For this review, take the finished solid that the model builds, in its own axes (mm). Give positions to 0.01 mm unless a question says otherwise; leave off trailing zeros. Loops run counter-clockwise (first coordinate to the right, second up) from the corner with the lowest first, then second, coordinate; pieces in that order, holes last. Notation, with made-up numbers: (57, 0.25) - (75, 0.25) arc R15 ccw to (75, 21.25) - close; hole circle Ø7 at (14.25, 68). An arc over 180 degrees is marked (long way). Answer as CSV lines item,"result".
from build123d import *

# Parameters (mm, degrees)
SKETCH1_R           = 2.6
BOSS_EXTRUDE1_DEPTH = 3.175


with BuildPart() as part:
    # Sketch1 → Boss-Extrude1 (new body)
    with BuildSketch(Plane(origin=(0, 0, 0), x_dir=(1, 0, 0), z_dir=(0, 1, 0))):
        Polygon((60, 0), (60, 20), (20, 60), (0, 60), (0, 0), align=None)
        with Locations((50, 10)):
            Circle(SKETCH1_R, mode=Mode.SUBTRACT)
        with Locations((10, 50)):
            Circle(SKETCH1_R, mode=Mode.SUBTRACT)
        with Locations((30, 10)):
            Circle(SKETCH1_R, mode=Mode.SUBTRACT)
        with Locations((10, 10)):
            Circle(SKETCH1_R, mode=Mode.SUBTRACT)
        with Locations((10, 30)):
            Circle(SKETCH1_R, mode=Mode.SUBTRACT)
    extrude(amount=BOSS_EXTRUDE1_DEPTH)


solid = part.part
1) Wall thickness on line 1 (X direction, y = 2, z = -10); line 2 (X direction, y = 2.45, z = -8.5); line 3 (Z direction, x = 50, y = 1.05): over which ranges is each line inside the solid? List them lowest first. Write a range as from..to.
From the geometry:
line 1,"x = 0..7.4, 12.6..27.4, 32.6..47.4, 52.6..60"
line 2,"x = 0..7.88, 12.12..27.88, 32.12..47.88, 52.12..60"
line 3,"z = -30..-12.6, -7.4..0"
2) Insertion check: P1, Ø1, axis at x = 25.5, y = 1.5, coming from the +Z side; P2, Ø4.5, axis at x = 10, z = -50, coming from the +Y side; P3, Ø1, axis at x = 50, y = 2.5, coming from the -Z side. Each pin has a flat end and moves straight along its axis. Give the tip position at first contact, or say it passes through.
From the geometry:
P1,"stops at z = 0"
P2,"passes through"
P3,"stops at z = -30.5"
3) Draft analysis for pull direction X (two halves, no side actions). For faces 1 (the flat face through (0, 2, -30)), 2 (the flat face through (60, 2, -10)), 3 (the cylindrical face through (11.4, 1.57, -32.19)), state which applies: pulls with the +X half, pulls with the -X half, needs draft (parallel to the pull), parting line crosses it, or undercut.
From the geometry:
face 1,"pulls with the -X half"
face 2,"pulls with the +X half"
face 3,"undercut"
4) Consider section B-B on z = -10. Write out the cut boundary in (x, y) (3 decimals).
From the geometry:
outline,"(0, 0) - (7.4, 0) - (7.4, 3.175) - (0, 3.175) - close; (12.6, 0) - (27.4, 0) - (27.4, 3.175) - (12.6, 3.175) - close; (32.6, 0) - (47.4, 0) - (47.4, 3.175) - (32.6, 3.175) - close; (52.6, 0) - (60, 0) - (60, 3.175) - (52.6, 3.175) - close"
5) Consider section C-C on y = 1.1. Write out the cut boundary in (x, z), and give its area (3 significant figures).
From the geometry:
outline,"(0, -60) - (20, -60) - (60, -20) - (60, 0) - (0, 0) - close; hole circle Ø5.2 at (10, -50); hole circle Ø5.2 at (10, -30); hole circle Ø5.2 at (10, -10); hole circle Ø5.2 at (30, -10); hole circle Ø5.2 at (50, -10)"
area,"2,690 mm^2"
6) Consider section A-A on x = 50. Write out the cut boundary in (y, z) (3 decimals), and give its area (3 significant figures).
From the geometry:
outline,"(0, -30) - (3.175, -30) - (3.175, -12.6) - (0, -12.6) - close; (0, -7.4) - (3.175, -7.4) - (3.175, 0) - (0, 0) - close"
area,"78.7 mm^2"
7) Consider section D-D on z = -30. Write out the cut boundary in (x, y) (3 decimals).
From the geometry:
outline,"(0, 0) - (7.4, 0) - (7.4, 3.175) - (0, 3.175) - close; (12.6, 0) - (50, 0) - (50, 3.175) - (12.6, 3.175) - close"
